Geometry: final body of the model. Coordinates: model frame, mm. Round coordinates to 2 decimals unless told otherwise and drop trailing zeros. Loops run counter-clockwise (first coordinate to the right, second up) from the corner with the lowest first, then second, coordinate; pieces in that order, holes last. Notation, with made-up numbers: (51, -27) -> (101, -27) arc R8 ccw to (101, -12) -> close; hole circle Ø10 at (22.5, 2.5). An arc over 180 degrees is marked (long way). Answer in a Markdown table with one row per item.
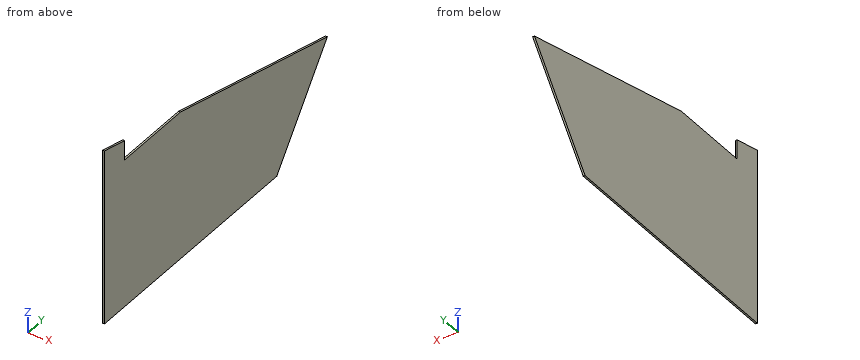
```python
from build123d import *

# Parameters (mm, degrees)
F1_DEPTH = 4.7625
F3_DEPTH = 4.7635
F5_DEPTH = 4.7635


with BuildPart() as f1:
    # F0 (on Right) → F1 (new body)
    with BuildSketch(Plane.YZ):
        Polygon((0, 457.2), (0, 0), (838.2, 0), (838.2, 254), align=None)
    extrude(amount=F1_DEPTH)

    # F2 (on face) → F3 (cut, through all)
    with BuildSketch(Plane(origin=(0, 0, 0), x_dir=(0, -1, 0), z_dir=(-1, 0, 0))):
        Polygon((-76.2, 387.927273), (-76.2, 438.727273), (-285.75, 387.927273), align=None)
    extrude(amount=-F3_DEPTH, mode=Mode.SUBTRACT)

    # F4 (on face) → F5 (cut, through all)
    with BuildSketch(Plane.YZ.offset(4.7625)):
        Polygon((838.2, 0), (838.2, 254), (647.7, 0), align=None)
    extrude(amount=-F5_DEPTH, mode=Mode.SUBTRACT)


solid = f1.part
```
Item 1: Cut plane A-A (x = 3.2). Output: boundary loops of the cut face in (y, z), then the cut area to 3 significant figures.
Answer:
| item | result |
|---|---|
| outline | (0, 0) -> (647.7, 0) -> (838.2, 254) -> (285.75, 387.93) -> (76.2, 387.93) -> (76.2, 438.73) -> (0, 457.2) -> close |
| area | 269,000 mm² |
Item 2: Line query: probe 1 along Z at (x, y) = (0.7, 246); probe 2 along Y at (x, z) = (1.2, 106); probe 3 along Y at (x, z) = (2.65, 24). Output: solid intervals per line, ascending. Write a range as [from, to].
Answer:
| item | result |
|---|---|
| probe 1 | z = [0, 387.93] |
| probe 2 | y = [0, 727.2] |
| probe 3 | y = [0, 665.7] |
Item 3: Cut plane C-C (y = 111). Output: boundary loops of the cut face in (x, z), then the cut area to 3 significant figures.
Answer:
| item | result |
|---|---|
| outline | (0, 0) -> (4.76, 0) -> (4.76, 387.93) -> (0, 387.93) -> close |
| area | 1,850 mm² |
Item 4: Pin query (flat end, axial travel): pin 1 Ø5 at (y, z) = (342, 194.5) entering from -X; pin 2 Ø1.4 at (x, y) = (2.5, 155.5) entering from +Z. Return the tip coordinate at first contact, or that it passes through.
Answer:
| item | result |
|---|---|
| pin 1 | stops at x = 0 |
| pin 2 | stops at z = 387.93 |
Item 5: Cut plane B-B (z = 428). Output: boundary loops of the cut face in (x, y).
Answer:
| item | result |
|---|---|
| outline | (0, 0) -> (4.76, 0) -> (4.76, 76.2) -> (0, 76.2) -> close |
